from build123d import *

# Parameters (mm, degrees)
SKETCH1_R           = 11
BOSS_EXTRUDE1_DEPTH = 2
SKETCH2_R           = 8.9
SKETCH2_R_2         = 7.9
BOSS_EXTRUDE2_DEPTH = 7
SKETCH3_R           = 1.65
CUT_EXTRUDE1_DEPTH  = 18.058722109
FILLET1_R           = 3
FILLET2_R           = 0.5


# Some blends are built 0.0001 mm under size
with BuildPart() as part:
    # Sketch1 → Boss-Extrude1 (new body)
    with BuildSketch(Plane(origin=(0, 0, 0), x_dir=(1, 0, 0), z_dir=(0, 1, 0))):
        with Locations(Location((0, 0, 0), (0, 0, 270))):
            Circle(SKETCH1_R)
    extrude(amount=BOSS_EXTRUDE1_DEPTH)

    # Sketch2 → Boss-Extrude2 (add)
    with BuildSketch(Plane(origin=(0, 2, 0), x_dir=(1, 0, 0), z_dir=(0, 1, 0))):
        with Locations(Location((0, 0, 0), (0, 0, 270))):
            Circle(SKETCH2_R)
        with Locations(Location((0, 0, 0), (0, 0, 270))):
            Circle(SKETCH2_R_2, mode=Mode.SUBTRACT)
    extrude(amount=BOSS_EXTRUDE2_DEPTH)

    # Sketch3 → Cut-Extrude1 (cut, through all)
    with BuildSketch(Plane(origin=(0, 2, 0), x_dir=(1, 0, 0), z_dir=(0, 1, 0))):
        with Locations(Location((0, 0, 0), (0, 0, 270))):
            Circle(SKETCH3_R)
    extrude(amount=-CUT_EXTRUDE1_DEPTH, mode=Mode.SUBTRACT)

    # Fillet1
    # the kernel refuses this fillet: 3 mm, written as the material it takes off along each edge
    with BuildSketch(Plane(origin=(0, 0, 0), x_dir=(0, 0, 1), z_dir=(-1, 0, 0))) as fillet1_piece_1:
        with BuildLine():
            CenterArc((8.171572875, 3), FILLET1_R, 270, 70.528779366)
            Line((8.171572875, 0), (8.171572875, -0.06))
            Line((8.171572875, -0.06), (11, -0.06))
            Line((11, -0.06), (11.06, 0))
            ThreePointArc((11.06, 0), (11.06, 1), (11.056568542, 1.98))
            Line((11.056568542, 1.98), (11, 2))
        make_face()
    revolve(axis=Axis((0, 0, 0), (0, 1, 0)), mode=Mode.SUBTRACT)

    # Fillet2
    fillet2_edges = [part.edges().sort_by_distance(p)[0] for p in [
        (0, 9, -8.9),
        (0, 9, -7.9),
    ]]
    fillet(fillet2_edges, radius=FILLET2_R - 0.0001)  # a hair under: the kernel refuses the full size


solid = part.part
Model file for the job. Use its own axes, mm. A direction names the side the tool comes from. Give positions to 0.01 mm unless a question says otherwise; leave off trailing zeros. Use a Markdown table: item, result. Add a question column.
(1) Drop flat-ended pins along their axis: pin 1 Ø1.5 at (x, y) = (-8, 3.5) entering from -Z; pin 2 Ø3 at (x, y) = (0.5, 6.5) entering from -Z; pin 3 Ø5 at (y, z) = (8, 5.5) entering from -X; pin 4 Ø2 at (x, z) = (0, 0) entering from -Y. Give the stop position or say it passes through.
(2) Tool access for faces 5 (the flat face through (2, 2, 0)), 6 (the flat face through (0, 0, 2)): list every direction of +Z, -Z, +X, -X, +Y, -Y with a clear straight run to the whole face (end or side of a thin tool).
(3) Mould opens along Z. For faces 1 (the cylindrical face through (6.015, 5.205, -6.56)), 2 (the flat face through (-9, 2, -1)), 3 (the cylindrical face through (5.34, 5.2, -5.82)), 4 (the cylindrical face through (-1, 1.01, -1.31)) say: +Z half, -Z half, draft (parallel to the pull), parting line (faces both ways), or undercut.
(4) Wall check: line 1 along X through (y, z) = (8.5, -0.25); line 2 along Y through (x, z) = (-0.5, -2.5); line 3 along Z through (x, y) = (-5.25, 6.5). Give the ranges that are in metal, low to high.
Filled sheet:
| question | item | result |
|---|---|---|
| 1 | pin 1 | z = -5.16 |
| 1 | pin 2 | z = -8.9 |
| 1 | pin 3 | x = -8.38 |
| 1 | pin 4 | through |
| 2 | face 5 | +Y |
| 2 | face 6 | +Z, -Z, +X, -X, -Y |
| 3 | face 1 | parting line |
| 3 | face 2 | draft |
| 3 | face 3 | undercut |
| 3 | face 4 | undercut |
| 4 | line 1 | -8.9 to -7.9, 7.9 to 8.9 |
| 4 | line 2 | 0 to 2 |
| 4 | line 3 | -7.19 to -5.9, 5.9 to 7.19 |
